Geometry check sheet. Reference: the model listing, model coordinates, mm. Face numbers are marked on the shaded views. A direction names the side the tool comes from. Round coordinates to 2 decimals unless told otherwise and drop trailing zeros. Write each loop counter-clockwise with the first axis right and the second up, starting at its lowest first coordinate (ties: lowest second). Pieces come first, ordered by that corner, then holes. Notation, with made-up numbers: M 82.25,56 L 132.25,56 A23 cw 132.25,93 Z; hole C -39.5,-1 d9. An arc over 180 degrees is marked long. One line per item, written item: value. Start each with the question number.
1. Section check D-D (x = -1). Record the boundary of the cut face in (y, z).
2. Release check for a two-part mould opening along X. For the marked faces 1, 2 and 3 record: pulls with the +X half, pulls with the -X half, needs draft (parallel to the pull), parting line crosses it, or undercut.
3. Section check B-B (x = 45). Record the boundary of the cut face in (y, z).
4. Depth check by flat-ended pin: P1, Ø5, axis at x = 13.5, z = 0.5, coming from the +Y side; P2, Ø5, axis at y = 31.5, z = -5.5, coming from the +X side; P3, Ø1.5, axis at x = 39, y = 7.5, coming from the -Z side; P4, Ø10, axis at x = 45, z = 0, coming from the +Y side. Enter the tip coordinate at first touch or a pass-through.
5. Scan lines: probe 1 along X at (y, z) = (2, 0); probe 2 along Z at (x, y) = (-34, 35); probe 3 along X at (y, z) = (8, 10.5). Record each from-to range of solid material in increasing order. Write a range as [from, to].
6. Access from +Z, -Z, +X, -X, +Y, -Y to the whole of each face (thin tool, end or side, straight path). Record for the marked faces 4, 5 and 6.
7. Section check A-A (z = -1). Record the boundary of the cut face in (x, y), and give its area (3 significant figures).
8. Section check C-C (z = 7.5). Record the boundary of the cut face in (x, y).
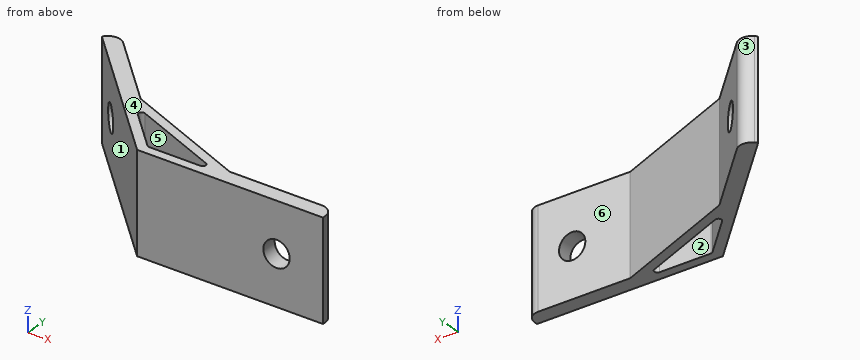
from build123d import *

# Parameters (mm, degrees)
EXTRUDE_1_DEPTH     = 16
SKETCH_2_R          = 4.25
CUT_EXTRUDE_1_DEPTH = 5
SKETCH_3_R          = 4.25
CUT_EXTRUDE_2_DEPTH = 5
FILLET_1_R          = 4
FILLET_2_R          = 1


with BuildPart() as part:
    # Эскиз1 → Бобышка-Вытянуть1 (new body, symmetric)
    with BuildSketch(Plane.XY):
        Polygon((0, 0), (-42.426406871, 42.426406871), (-38.890872965, 45.961940777), (-15.028558569, 22.099626381), (26.253591352, 5), (60, 5), (60, 0), align=None)
        Polygon((-14.313708499, 18.556349186), (23.242640687, 3), (1.242640687, 3), align=None, mode=Mode.SUBTRACT)
    extrude(amount=EXTRUDE_1_DEPTH, both=True)

    # Эскиз2 → Вырез-Вытянуть1 (cut)
    with BuildSketch(Plane(origin=(0, 0, 0), x_dir=(0, 0, 1), z_dir=(-0.707106781, -0.707106781, 0))):
        with Locations(Location((0, 45, 0), (0, 0, 270))):  # turned: the seam where the file's is
            Circle(SKETCH_2_R)
    extrude(amount=-CUT_EXTRUDE_1_DEPTH, mode=Mode.SUBTRACT)

    # Эскиз3 → Вырез-Вытянуть2 (cut)
    with BuildSketch(Plane.XZ):
        with Locations(Location((45, 0, 0), (0, 0, 270))):  # turned: the seam where the file's is
            Circle(SKETCH_3_R)
    extrude(amount=-CUT_EXTRUDE_2_DEPTH, mode=Mode.SUBTRACT)

    # Скругление1
    fillet_1_edges = [part.edges().sort_by_distance(p)[0] for p in [
        (-38.890872965, 45.961940777, 0),
        (60, 5, 0),
    ]]
    fillet(fillet_1_edges, radius=FILLET_1_R)

    # Скругление2
    fillet_2_edges = [part.edges().sort_by_distance(p)[0] for p in [
        (-14.313708499, 18.556349186, 0),
        (1.242640687, 3, 0),
        (23.242640687, 3, 0),
    ]]
    fillet(fillet_2_edges, radius=FILLET_2_R)


solid = part.part
Result sheet:
1. outline: M 1,-16 L 5.24,-16 L 5.24,16 L 1,16 Z; M 13.04,-16 L 16.29,-16 L 16.29,16 L 13.04,16 Z
2. face 1: pulls with the -X half
2. face 2: undercut
2. face 3: parting line crosses it
3. outline: M 0,-16 L 5,-16 L 5,-4.25 L 0,-4.25 Z; M 0,4.25 L 5,4.25 L 5,16 L 0,16 Z
4. P1: stops at y = 11.32
4. P2: stops at x = -21.93
4. P3: passes through
4. P4: stops at y = 5
5. probe 1: x = [-2, 40.75], [49.25, 59.87]
5. probe 2: z = [-16, -1.92], [1.92, 16]
5. probe 3: x = [-8, -3.76], [11.17, 19.01]
6. face 4: +Z, +X, -X, +Y, -Y
6. face 5: +Z, -Z
6. face 6: +Z, -Z, +X, +Y
7. outline: M -42.43,42.43 L -34.74,34.74 L -31.21,38.28 L -36.06,43.13 A4 ccw -41.72,43.13 Z; M -28.9,28.9 L 0,0 L 40.87,0 L 40.87,5 L 26.25,5 L -15.03,22.1 L -25.36,32.43 Z; M 49.13,0 L 60,0 L 60,1 A4 ccw 56,5 L 49.13,5 Z; hole M -10.76,15 L 0.95,3.29 A1 ccw 1.66,3 L 18.22,3 A1 ccw 18.6,4.92 L -9.67,16.63 A1 ccw Z
7. area: 543 mm2
8. outline: M -42.43,42.43 L 0,0 L 60,0 L 60,1 A4 ccw 56,5 L 26.25,5 L -15.03,22.1 L -36.06,43.13 A4 ccw -41.72,43.13 Z; hole M -10.76,15 L 0.95,3.29 A1 ccw 1.66,3 L 18.22,3 A1 ccw 18.6,4.92 L -9.67,16.63 A1 ccw Z
